Verification items for the finished model (mm, model axes). Face numbers are marked on the shaded views. A direction names the side the tool comes from. Round coordinates to 2 decimals unless told otherwise and drop trailing zeros. Write each loop counter-clockwise with the first axis right and the second up, starting at its lowest first coordinate (ties: lowest second). Pieces come first, ordered by that corner, then holes. Notation, with made-up numbers: M 61,56 L 79,56 A6 ccw 79,62 Z; hole C 33,-27.75 d1. An arc over 180 degrees is marked long. Answer in a Markdown table with one row per item. Add a question column.
1. Sectioned sample at B-B on z = 10.5. Record the cut outline in (x, y).
2. Material ranges on probe 1 along Y at (x, z) = (14, 12); probe 2 along Z at (x, y) = (-10.5, 18); probe 3 along X at (y, z) = (-1, 7.25), recorded low to high.
3. Go/stop test with flat-tipped pins: pin 1 Ø0.8 at (x, y) = (-17.5, -3) entering from -Z; pin 2 Ø3 at (y, z) = (5, 20) entering from -X; pin 3 Ø8 at (x, z) = (3, 22.5) entering from -Y. Record where each tip stops, or that it passes through.
4. Sectioned sample at D-D on x = -2. Record the cut outline in (y, z), plus the area to 3 significant figures.
5. Draft check along Y on the marked faces 1, 2 and 3. Enter one of: pulls with the +Y half, pulls with the -Y half, needs draft (parallel to the pull), parting line crosses it, or undercut.
6. Sectioned sample at A-A on y = 2.5. Record the cut outline in (x, z).
7. Sectioned sample at C-C on y = 6. Record the cut outline in (x, z).
8. Set-up check for the marked faces 4 and 5: record each of +Z, -Z, +X, -X, +Y, -Y from which the full face is reachable in a straight line by a thin tool's end or side.
```python
from build123d import *

# Parameters (mm, degrees)
SKETCH_2_R          = 1.75
EXTRUDE_1_DEPTH     = 25
SKETCH_3_W          = 1
SKETCH_3_H          = 8
CUT_EXTRUDE_1_DEPTH = 1
SKETCH_4_R          = 2
CUT_EXTRUDE_2_DEPTH = 9
SKETCH_5_W          = 3
SKETCH_5_H          = 5.5
CUT_EXTRUDE_3_DEPTH = 33


with BuildPart() as part:
    # Эскиз2 → Бобышка-Вытянуть1 (new body)
    with BuildSketch(Plane.XY):
        with BuildLine():
            Line((8, 0), (8, -12))
            Line((8, -12), (20, -12))
            Line((20, -12), (20, 20))
            Line((20, 20), (-18, 20))
            Line((-18, 20), (-18, -12))
            Line((-18, -12), (0, -12))
            Line((0, -12), (0, -8))
            ThreePointArc((0, -8), (-5.656854249, 5.656854249), (8, 0))
        make_face()
        with Locations((1, 14)):
            Circle(SKETCH_2_R, mode=Mode.SUBTRACT)
        with Locations((14, -7)):
            Circle(SKETCH_2_R, mode=Mode.SUBTRACT)
        with Locations((14, 14)):
            Circle(SKETCH_2_R, mode=Mode.SUBTRACT)
    extrude(amount=EXTRUDE_1_DEPTH)

    # Эскиз3 → Вырез-Вытянуть1 (cut)
    with BuildSketch(Plane.ZY.offset(18)):
        with Locations((0.5, -2)):
            Rectangle(SKETCH_3_W, SKETCH_3_H)
        with Locations((2.5, -2)):
            Rectangle(SKETCH_3_W, SKETCH_3_H)
        with Locations((4.5, -2)):
            Rectangle(SKETCH_3_W, SKETCH_3_H)
        with Locations((6.5, -2)):
            Rectangle(SKETCH_3_W, SKETCH_3_H)
        with Locations((8.5, -2)):
            Rectangle(SKETCH_3_W, SKETCH_3_H)
        with Locations((10.5, -2)):
            Rectangle(SKETCH_3_W, SKETCH_3_H)
        with Locations((12.5, -2)):
            Rectangle(SKETCH_3_W, SKETCH_3_H)
        with Locations((14.5, -2)):
            Rectangle(SKETCH_3_W, SKETCH_3_H)
        with Locations((16.5, -2)):
            Rectangle(SKETCH_3_W, SKETCH_3_H)
        with Locations((18.5, -2)):
            Rectangle(SKETCH_3_W, SKETCH_3_H)
        with Locations((20.5, -2)):
            Rectangle(SKETCH_3_W, SKETCH_3_H)
        with Locations((22.5, -2)):
            Rectangle(SKETCH_3_W, SKETCH_3_H)
        with Locations((24.5, -2)):
            Rectangle(SKETCH_3_W, SKETCH_3_H)
    extrude(amount=-CUT_EXTRUDE_1_DEPTH, mode=Mode.SUBTRACT)

    # Эскиз4 → Вырез-Вытянуть2 (cut)
    with BuildSketch(Plane.ZY.offset(18)):
        with Locations((5, 5)):
            Circle(SKETCH_4_R)
        with Locations((20, 5)):
            Circle(SKETCH_4_R)
        with Locations((20, -9)):
            Circle(SKETCH_4_R)
        with Locations((5, -9)):
            Circle(SKETCH_4_R)
    extrude(amount=-CUT_EXTRUDE_2_DEPTH, mode=Mode.SUBTRACT)

    # Эскиз5 → Вырез-Вытянуть3 (cut, through all)
    with BuildSketch(Plane.XZ.offset(12)):
        with Locations((-10.5, 5)):
            Rectangle(SKETCH_5_W, SKETCH_5_H)
        with Locations((-10.5, 20)):
            Rectangle(SKETCH_5_W, SKETCH_5_H)
    extrude(amount=-CUT_EXTRUDE_3_DEPTH, mode=Mode.SUBTRACT)


solid = part.part
```
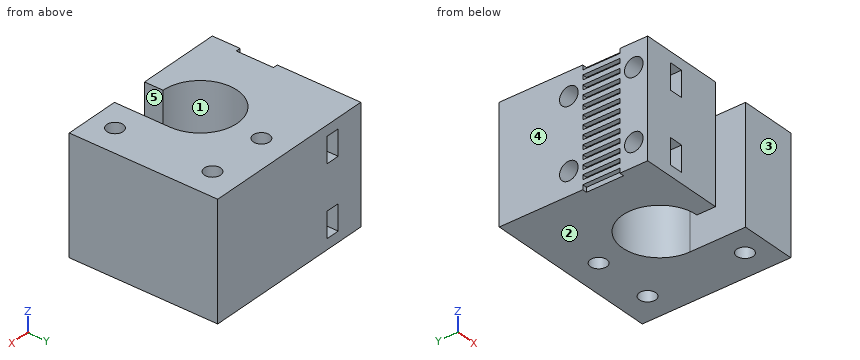
Geometry check:
| question | item | result |
|---|---|---|
| 1 | outline | M -18,-12 L 0,-12 L 0,-8 A8 cw long 8,0 L 8,-12 L 20,-12 L 20,20 L -18,20 L -18,2 L -17,2 L -17,-6 L -18,-6 Z; hole C 1,14 d3.5; hole C 14,-7 d3.5; hole C 14,14 d3.5 |
| 2 | probe 1 | y = -12 to -8.75, -5.25 to 12.25, 15.75 to 20 |
| 2 | probe 2 | z = 0 to 2.25, 7.75 to 17.25, 22.75 to 25 |
| 2 | probe 3 | x = -18 to -12, -9 to -7.94, 8 to 20 |
| 3 | pin 1 | stops at z = 1 |
| 3 | pin 2 | stops at x = -9 |
| 3 | pin 3 | stops at y = -12 |
| 4 | outline | M -12,0 L -7.75,0 L -7.75,25 L -12,25 Z; M 7.75,0 L 20,0 L 20,25 L 7.75,25 Z |
| 4 | area | 413 mm2 |
| 5 | face 1 | undercut |
| 5 | face 2 | needs draft |
| 5 | face 3 | pulls with the -Y half |
| 6 | outline | M -18,0 L -7.6,0 L -7.6,25 L -18,25 Z; M 7.6,0 L 20,0 L 20,25 L 7.6,25 Z; hole M -12,2.25 L -9,2.25 L -9,7.75 L -12,7.75 Z; hole M -12,17.25 L -9,17.25 L -9,22.75 L -12,22.75 Z |
| 7 | outline | M -18,0 L -5.29,0 L -5.29,25 L -18,25 L -18,21.73 L -12,21.73 L -12,22.75 L -9,22.75 L -9,17.25 L -12,17.25 L -12,18.27 L -18,18.27 L -18,6.73 L -12,6.73 L -12,7.75 L -9,7.75 L -9,2.25 L -12,2.25 L -12,3.27 L -18,3.27 Z; M 5.29,0 L 20,0 L 20,25 L 5.29,25 Z |
| 8 | face 4 | +Z, -Z, -X, +Y, -Y |
| 8 | face 5 | +Z, -Z, -Y |
